from build123d import *

# Parameters (mm, degrees)
SKETCH_1_W          = 138
SKETCH_1_H          = 28
EXTRUDE_1_DEPTH     = 8
SKETCH_2_W          = 103
SKETCH_2_H          = 8
EXTRUDE_2_DEPTH     = 97
SKETCH_3_W          = 138
SKETCH_3_H          = 28
EXTRUDE_3_DEPTH     = 8
SKETCH_4_R          = 2.5
CUT_EXTRUDE_1_DEPTH = 5
SKETCH_5_R          = 2.5
CUT_EXTRUDE_2_DEPTH = 5


with BuildPart() as part:
    # 草图1 → 凸台-拉伸1 (new body)
    with BuildSketch(Plane(origin=(0, 0, 0), x_dir=(0, 0, -1), z_dir=(1, 0, 0))):
        Rectangle(SKETCH_1_W, SKETCH_1_H)
    extrude(amount=EXTRUDE_1_DEPTH)

    # 草图2 → 凸台-拉伸2 (add)
    with BuildSketch(Plane.ZY):
        with Locations((0.5, -10)):
            Rectangle(SKETCH_2_W, SKETCH_2_H)
    extrude(amount=EXTRUDE_2_DEPTH)

    # 草图3 → 凸台-拉伸3 (add)
    with BuildSketch(Plane.ZY.offset(97)):
        with Locations((0.070183463, -0.989678925)):
            Rectangle(SKETCH_3_W, SKETCH_3_H)
    extrude(amount=EXTRUDE_3_DEPTH)

    # 草图4 → 切除-拉伸1 (cut)
    with BuildSketch(Plane.XY.offset(69.070183463)):
        with Locations((-101.073349409, 9.731398078)):
            Circle(SKETCH_4_R)
        with Locations((3.926650591, 9.731398078)):
            Circle(SKETCH_4_R)
        with Locations((3.926650591, -10.268601922)):
            Circle(SKETCH_4_R)
        with Locations((-101.073349409, -10.268601922)):
            Circle(SKETCH_4_R)
    extrude(amount=-CUT_EXTRUDE_1_DEPTH, mode=Mode.SUBTRACT)

    # 草图5 → 切除-拉伸2 (cut)
    with BuildSketch(Plane(origin=(0, 0, -69), x_dir=(-1, 0, 0), z_dir=(0, 0, -1))):
        with Locations((-4, 10)):
            Circle(SKETCH_5_R)
        with Locations((101, 10)):
            Circle(SKETCH_5_R)
        with Locations((101, -10)):
            Circle(SKETCH_5_R)
        with Locations((-4, -10)):
            Circle(SKETCH_5_R)
    extrude(amount=-CUT_EXTRUDE_2_DEPTH, mode=Mode.SUBTRACT)


solid = part.part
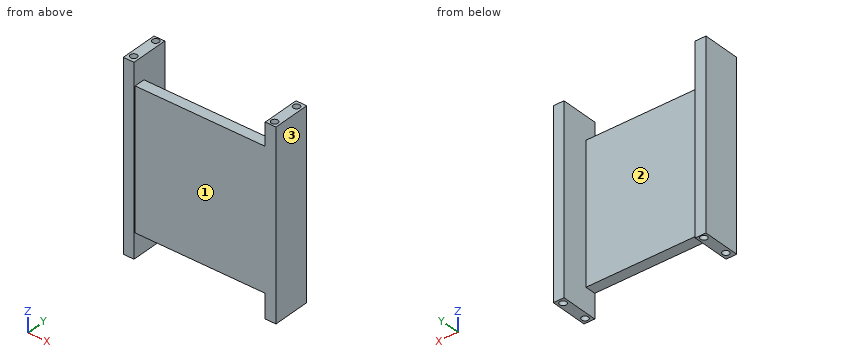
Can you work these out from the model? Positions are in its coordinate system, mm. Face numbers are marked on the shaded views. A direction names the side the tool comes from. Coordinates: 2 decimals unless noted, no trailing zeros. Loops run counter-clockwise (first coordinate to the right, second up) from the corner with the lowest first, then second, coordinate; pieces in that order, holes last. Notation, with made-up numbers: M 55.5,-10.75 L 83.5,-10.75 A31 ccw 83.5,21.25 Z; hole C 68.25,-8.5 d3. An arc over 180 degrees is marked long. Answer as CSV lines item,"result". Start each with the question number.
1. Suppose I cut it at A-A, the plane y = 5. List the corners of the cut face in (x, z) for me, plus the area to 3 significant figures.
2. For the marked faces 1, 2 and 3, which set-ups out of +Z, -Z, +X, -X, +Y, -Y let a thin tool reach every point of the face, with its end or its side?
3. For pin 1 Ø8 at (x, z) = (-40, 24) entering from +Y; pin 2 Ø3 at (x, y) = (-101, -10) entering from +Z; pin 3 Ø5.5 at (x, y) = (4.5, -10) entering from -Z; pin 4 Ø5 at (x, y) = (-14, -7.5) entering from +Z, each with a flat end and sliding along its axis, tell me the tip position at first contact or that it passes through.
4. If I drill on probe 1 along Y at (x, z) = (-101, -65.9); probe 2 along X at (y, z) = (5.25, -56.5); probe 3 along Z at (x, y) = (-57.5, -10), over which ranges is the centre line in solid material (lowest first)? Write a range as [from, to].
5. Suppose I cut it at C-C, the plane x = 4. List the corners of the cut face in (y, z) for me.
6. Suppose I cut it at B-B, the plane z = 6. List the corners of the cut face in (x, y) for me.
Output:
1,outline,"M -105,-68.93 L -97,-68.93 L -97,69.07 L -105,69.07 Z; M 0,-69 L 8,-69 L 8,69 L 0,69 Z"
1,area,"2,210 mm^2"
2,face 1,"+Z, -Z, +X, -Y"
2,face 2,"+Z, -Z, +Y"
2,face 3,"+Z, -Z, +X, +Y, -Y"
3,pin 1,"stops at y = -6"
3,pin 2,"stops at z = 64.07"
3,pin 3,"stops at z = -69"
3,pin 4,"stops at z = 52"
4,probe 1,"y = [-14.99, -12.5], [-7.5, 7.5], [12.5, 13.01]"
4,probe 2,"x = [-105, -97], [0, 8]"
4,probe 3,"z = [-51, 52]"
5,outline,"M -14,-69 L -12.5,-69 L -12.5,-64 L -7.5,-64 L -7.5,-69 L 7.5,-69 L 7.5,-64 L 12.5,-64 L 12.5,-69 L 14,-69 L 14,69 L 12.23,69 L 12.23,64.07 L 7.23,64.07 L 7.23,69 L -7.77,69 L -7.77,64.07 L -12.77,64.07 L -12.77,69 L -14,69 Z"
6,outline,"M -105,-14.99 L -97,-14.99 L -97,-14 L 8,-14 L 8,14 L 0,14 L 0,-6 L -97,-6 L -97,13.01 L -105,13.01 Z"
